Part print with two shaded views. Sizes in mm from the minimum x, y, z corner. Round coordinates to 2 decimals unless told otherwise and drop trailing zeros. Write each loop counter-clockwise with the first axis right and the second up, starting at its lowest first coordinate (ties: lowest second). Pieces come first, ordered by that corner, then holes. Notation, with made-up numbers: (50, -21.75) -> (102, -21.75) arc R27 ccw to (102, 14.25) -> close; hole circle Ø8 at (19, 17.25). An arc over 180 degrees is marked (long way). Answer in a Markdown table with one row per item. Add a question column.
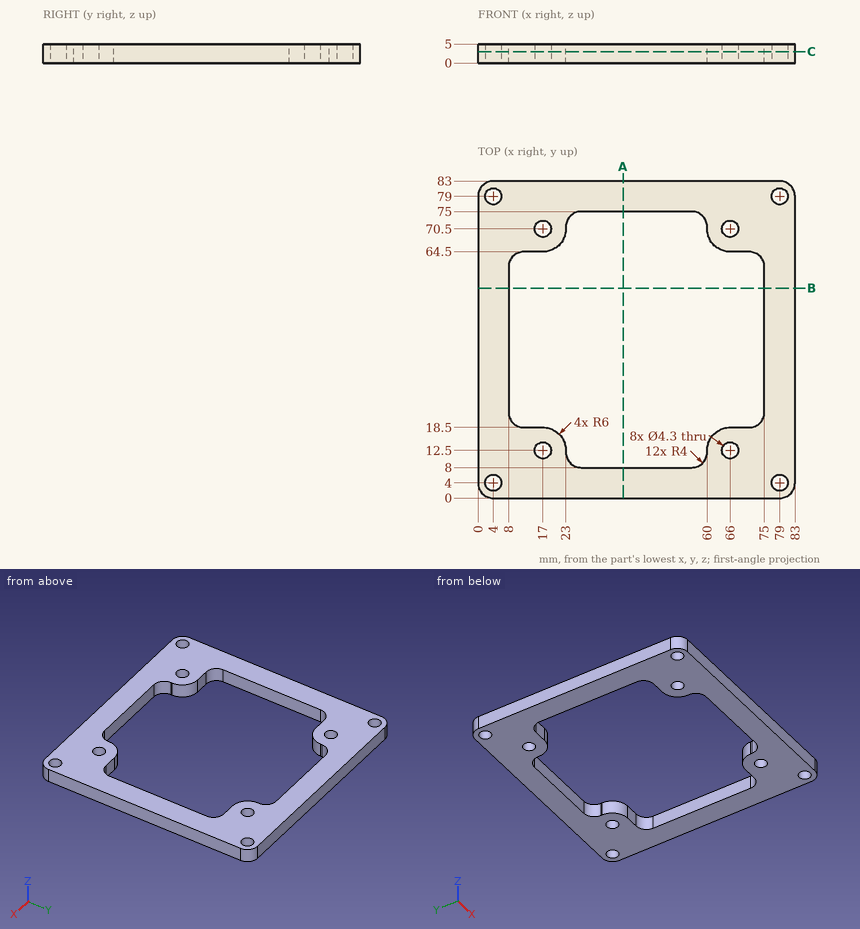
Item 1: Saw through at C-C on z = 3. Count the separate pieces of the cut face and the enclosed holes in it, then the cut area to 3 significant figures.
Item 2: Drill centre lines: probe 1 along Y at (x, z) = (79, 3.85); probe 2 along Y at (x, z) = (47, 3); probe 3 along X at (y, z) = (71.5, 4.8). Where is each one in solid material? Low to high.
Item 3: Saw through at A-A on x = 38. Give the cut face in (y, z).
Item 4: Pin check, flat tips, straight feed: pin 1 (7 mm diameter, centred on x = 66, y = 12.5, fed in from +Z); pin 2 (2.5 mm diameter, centred on x = 79, y = 4, fed in from +Z). Stop position of each tip, or through.
Recorded:
| question | item | result |
|---|---|---|
| 1 | separate pieces | 1 |
| 1 | enclosed holes | 9 |
| 1 | area | 2,900 mm2 |
| 2 | probe 1 | 0 to 1.85, 6.15 to 76.85, 81.15 to 83 |
| 2 | probe 2 | 0 to 8, 75 to 83 |
| 2 | probe 3 | 0 to 15.1, 18.9 to 23.03, 59.97 to 64.1, 67.9 to 83 |
| 3 | outline | (0, 0) -> (8, 0) -> (8, 5) -> (0, 5) -> close; (75, 0) -> (83, 0) -> (83, 5) -> (75, 5) -> close |
| 4 | pin 1 | z = 5 |
| 4 | pin 2 | through |
